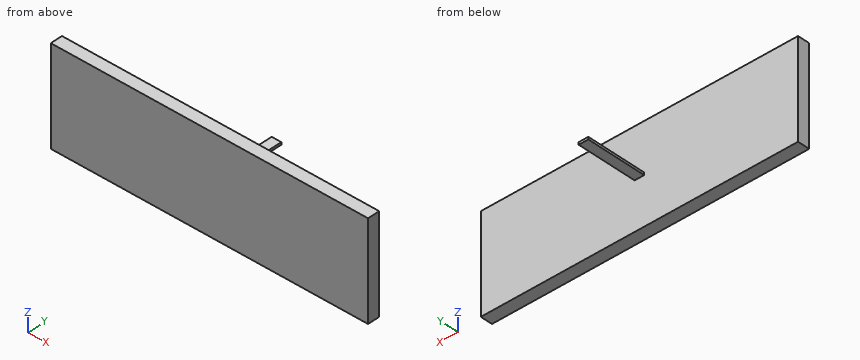
from build123d import *

# Parameters (mm, degrees)
SKETCH1_W                = 132
SKETCH1_H                = 40
BOSS_EXTRUDE1_DEPTH      = 5
SKETCH2_W                = 4
SKETCH2_H                = 30
BOSS_EXTRUDE2_DEPTH      = 0.5
BOSS_EXTRUDE2_DEPTH_BACK = 0.5


with BuildPart() as part:
    # Sketch1 → Boss-Extrude1 (new body)
    with BuildSketch(Plane(origin=(0, 0, 0), x_dir=(1, 0, 0), z_dir=(0, 1, 0))):
        Rectangle(SKETCH1_W, SKETCH1_H)
    extrude(amount=BOSS_EXTRUDE1_DEPTH)

    # Sketch2 → Boss-Extrude2 (add, two sides)
    with BuildSketch(Plane.XY) as boss_extrude2_sk:
        with Locations((0, 15)):
            Rectangle(SKETCH2_W, SKETCH2_H)
    extrude(amount=BOSS_EXTRUDE2_DEPTH)
    extrude(boss_extrude2_sk.sketch, amount=-BOSS_EXTRUDE2_DEPTH_BACK)


solid = part.part
The listing builds one solid part. Answer for the finished solid, in the listing's coordinates (mm). Coordinates: 2 decimals unless noted, no trailing zeros. Loops run counter-clockwise (first coordinate to the right, second up) from the corner with the lowest first, then second, coordinate; pieces in that order, holes last. Notation, with made-up numbers: M -8,84 L 2,84 A15 cw 2,109 Z; hole C 2.5,26 d5. An arc over 180 degrees is marked long. Answer in a Markdown table with one row per item.
1) Given pin 1 (12 mm diameter, centred on x = 7, y = 21.5, fed in from -Z); pin 2 (8 mm diameter, centred on x = -34.5, z = 4.5, fed in from +Y); pin 3 (3 mm diameter, centred on x = -0.5, y = 14.5, fed in from +Z), each flat-ended and moving along its own axis, determine where each tip first touches the part or whether it passes through.
Answers below:
| item | result |
|---|---|
| pin 1 | z = -0.5 |
| pin 2 | y = 5 |
| pin 3 | z = 0.5 |
2) Find section A-A (z = 3). Determine the outline of the cut face in (x, y), then the cut area to 3 significant figures.
Answers below:
| item | result |
|---|---|
| outline | M -66,0 L 66,0 L 66,5 L -66,5 Z |
| area | 660 mm^2 |
3) Find the intervals of material crossed by probe 1 along Y at (x, z) = (-48, -15); probe 2 along Z at (x, y) = (0, 5.25), in increasing order.
Answers below:
| item | result |
|---|---|
| probe 1 | 0 to 5 |
| probe 2 | -0.5 to 0.5 |
4) Find section B-B (y = 10.5). Determine the outline of the cut face in (x, z), then the cut area to 3 significant figures.
Answers below:
| item | result |
|---|---|
| outline | M -2,-0.5 L 2,-0.5 L 2,0.5 L -2,0.5 Z |
| area | 4.00 mm^2 |
